```python
from build123d import *

# Parameters (mm, degrees)
SKICA1_R                 = 30
SKICA1_R_2               = 5
P_IDAT_VYSUNUT_M1_DEPTH  = 5
ODEBRAT_VYSUNUT_M1_REACH = 7
SKICA2_R                 = 3
ZAOBLIT1_R               = 0.5


with BuildPart() as part:
    # Skica1 → Přidat vysunutím1 (new body)
    with BuildSketch(Plane(origin=(0, 0, 0), x_dir=(0, 0, -1), z_dir=(1, 0, 0))):
        Circle(SKICA1_R)
        Circle(SKICA1_R_2, mode=Mode.SUBTRACT)
    extrude(amount=P_IDAT_VYSUNUT_M1_DEPTH)

    # Skica2 → Odebrat vysunutím1 (cut, up to next)
    with BuildSketch(Plane.ZY, mode=Mode.PRIVATE) as odebrat_vysunut_m1_sk1:
        with Locations((0, -24)):
            Circle(SKICA2_R)
    odebrat_vysunut_m1_tool1 = extrude(odebrat_vysunut_m1_sk1.sketch, amount=-ODEBRAT_VYSUNUT_M1_REACH, mode=Mode.PRIVATE) & part.part
    add(odebrat_vysunut_m1_tool1.solids().sort_by_distance((0, -24, 0))[0], mode=Mode.SUBTRACT)

    # Zaoblit1
    zaoblit1_edges = [part.edges().sort_by_distance(p)[0] for p in [
        (0, 0, 30),
        (5, 0, 30),
    ]]
    fillet(zaoblit1_edges, radius=ZAOBLIT1_R)


solid = part.part
```
Can you work these out from the model? Positions are in its coordinate system, mm. Coordinates: 2 decimals unless noted, no trailing zeros. Write each loop counter-clockwise with the first axis right and the second up, starting at its lowest first coordinate (ties: lowest second). Pieces come first, ordered by that corner, then holes. Notation, with made-up numbers: M 18,63 L 26,63 A29 ccw 26,89 Z; hole C 14.5,14.5 d7. An arc over 180 degrees is marked long. Answer as CSV lines item,"result".
Item 1: Imagine slicing it at B-B on y = 0. List the corners of the cut face in (x, z) for me.
Geometry results:
outline,"M 0,-29.5 A0.5 ccw 0.5,-30 L 4.5,-30 A0.5 ccw 5,-29.5 L 5,-5 L 0,-5 Z; M 0,5 L 5,5 L 5,29.5 A0.5 ccw 4.5,30 L 0.5,30 A0.5 ccw 0,29.5 Z"
Item 2: We'd pull the mould along Y, two halves only. Please class faces 1 (the cylindrical face through (2.46, -4.88, 1.08)), 2 (the flat face through (5, 0, -6)), 3 (the cylindrical face through (2.47, 1.32, 29.97)), 4 (the cylindrical face through (2.46, -26.93, -0.65)): +Y half, -Y half, draft (parallel to the pull), parting line (faces both ways), or undercut.
Geometry results:
face 1,"undercut"
face 2,"draft"
face 3,"parting line"
face 4,"undercut"
Item 3: Imagine slicing it at C-C on x = 3.05. List the corners of the cut face in (y, z) for me, plus the area to 3 significant figures.
Geometry results:
outline,"C 0,0 d60; hole C -24,0 d6; hole C 0,0 d10"
area,"2,720 mm2"
Item 4: I'm going to push flat-ended pins straight in: P1, Ø1.5, axis at x = 2.5, y = -6, coming from the -Z side; P2, Ø3, axis at x = 2, z = -20, coming from the -Y side. Where does each tip first touch, or does it pass through?
Geometry results:
P1,"stops at z = -29.54"
P2,"stops at y = -23.62"
Item 5: Imagine slicing it at A-A on z = 0. List the corners of the cut face in (x, y) for me.
Geometry results:
outline,"M 0,-29.5 A0.5 ccw 0.5,-30 L 4.5,-30 A0.5 ccw 5,-29.5 L 5,-27 L 0,-27 Z; M 0,-21 L 5,-21 L 5,-5 L 0,-5 Z; M 0,5 L 5,5 L 5,29.5 A0.5 ccw 4.5,30 L 0.5,30 A0.5 ccw 0,29.5 Z"
Item 6: Please list where these lines run through material, in increasing order: line 1 along Y through (x, z) = (2.05, 0); line 2 along Y through (x, z) = (3.1, 4.5); line 3 along Z through (x, y) = (1.2, -26).
Geometry results:
line 1,"y = -30 to -27, -21 to -5, 5 to 30"
line 2,"y = -29.66 to -2.18, 2.18 to 29.66"
line 3,"z = -14.97 to -2.24, 2.24 to 14.97"
